Drawing for the job (mm, zero at the part's lowest x, y, z). A direction names the side the tool comes from. Coordinates: 2 decimals unless noted, no trailing zeros. Write each loop counter-clockwise with the first axis right and the second up, starting at its lowest first coordinate (ties: lowest second). Pieces come first, ordered by that corner, then holes. Notation, with made-up numbers: (1.5, 29) -> (27.5, 29) arc R18 cw to (27.5, 60) -> close; hole circle Ø4 at (-39.5, 30). An arc over 180 degrees is marked (long way). Write item = value, one per line. Start each with the question number.
Q1. Probe line 1 (Y direction, x = 24, z = 1.5); line 2 (Y direction, x = 13, z = 0.85); line 3 (X direction, y = 9.5, z = 1.4). List the from-to ranges inside material, lowest first.
Q2. Band-saw the part on C-C, the plane y = 12.25. List the corners of the cut face in (x, z).
Q3. Band-saw the part on B-B, the plane z = 2.45. List the corners of the cut face in (x, y), plus the area to 3 significant figures.
Q4. Pin check, flat tips, straight feed: P1, Ø8, axis at x = 13, y = 5, coming from the +Z side; P2, Ø1.6, axis at x = 11.5, z = 1.5, coming from the +Y side; P3, Ø1, axis at x = 9, z = 0.5, coming from the -Y side; P4, Ø1.7, axis at x = 24, y = 17, coming from the +Z side. Stop position of each tip, or through.
Q5. Band-saw the part on A-A, the plane x = 24. List the corners of the cut face in (y, z).
Q6. Pull direction Y, two halves, no side cores. Call the marked faces 3, 4 and 5: released by +Y, released by -Y, zero draft, split by the parting line, or undercut.
Q7. Tool access for the marked faces 1 and 2: list every direction of +Z, -Z, +X, -X, +Y, -Y with a clear straight run to the whole face (end or side of a thin tool).
Q8. Band-saw the part on D-D, the plane x = 17.5. List the corners of the cut face in (y, z), plus the area to 3 significant figures.
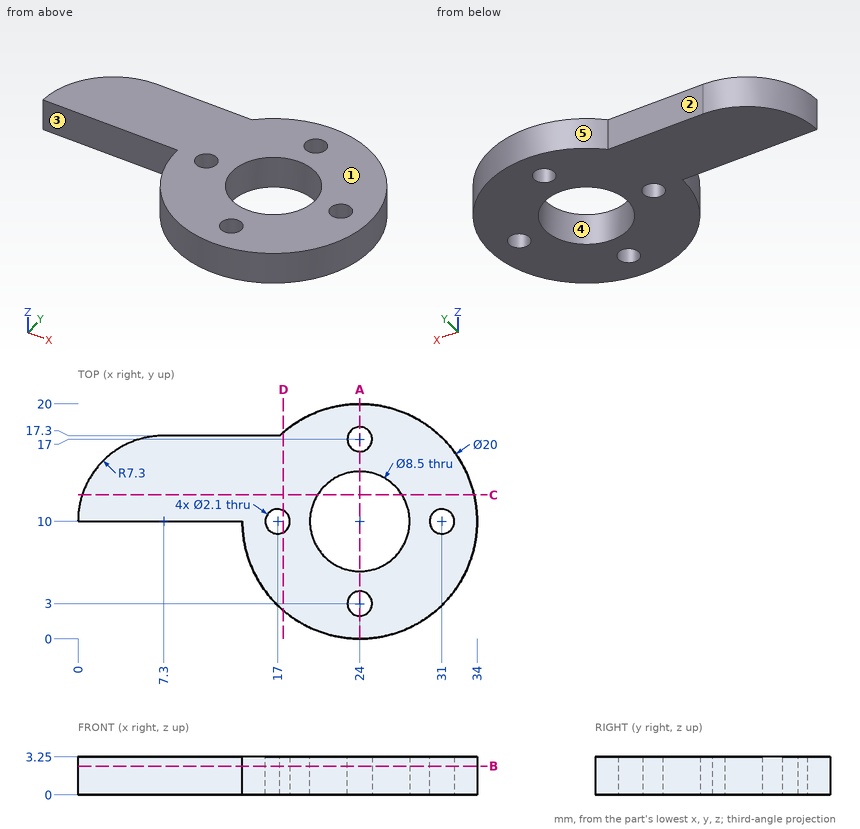
Ans:
q1.line_1 = 0 to 1.95, 4.05 to 5.75, 14.25 to 15.95, 18.05 to 20
q1.line_2 = 10 to 17.3
q1.line_3 = 14.01 to 16.08, 17.92 to 19.78, 28.22 to 30.08, 31.92 to 33.99
q2.outline = (0.36, 0) -> (20.39, 0) -> (20.39, 3.25) -> (0.36, 3.25) -> close; (27.61, 0) -> (33.74, 0) -> (33.74, 3.25) -> (27.61, 3.25) -> close
q3.outline = (0, 10) -> (14, 10) arc R10 ccw (long way) to (17.17, 17.3) -> (7.3, 17.3) arc R7.3 ccw to start; hole circle Ø2.1 at (17, 10); hole circle Ø8.5 at (24, 10); hole circle Ø2.1 at (24, 3); hole circle Ø2.1 at (24, 17); hole circle Ø2.1 at (31, 10)
q3.area = 341 mm2
q4.P1 = 3.25
q4.P2 = 17.3
q4.P3 = 10
q4.P4 = through
q5.outline = (0, 0) -> (1.95, 0) -> (1.95, 3.25) -> (0, 3.25) -> close; (4.05, 0) -> (5.75, 0) -> (5.75, 3.25) -> (4.05, 3.25) -> close; (14.25, 0) -> (15.95, 0) -> (15.95, 3.25) -> (14.25, 3.25) -> close; (18.05, 0) -> (20, 0) -> (20, 3.25) -> (18.05, 3.25) -> close
q6.face_3 = released by -Y
q6.face_4 = undercut
q6.face_5 = split by the parting line
q7.face_1 = +Z, +X, -X, +Y, -Y
q7.face_2 = +Z, -Z, -X, +Y
q8.outline = (2.4, 0) -> (9.08, 0) -> (9.08, 3.25) -> (2.4, 3.25) -> close; (10.92, 0) -> (17.6, 0) -> (17.6, 3.25) -> (10.92, 3.25) -> close
q8.area = 43.4 mm2
